```python
from build123d import *

# Parameters (mm, degrees)
CROQUIS1_W              = 400
CROQUIS1_H              = 250
SALIENTE_EXTRUIR1_DEPTH = 200
CORTAR_EXTRUIR1_DEPTH   = 115
SALIENTE_EXTRUIR2_DEPTH = 100
CHAFL_N1_SIZE           = 100
CHAFL_N1_SIZE2          = 127.994163219
CHAFL_N2_SIZE           = 127.994163219
CHAFL_N2_SIZE_2         = 100


with BuildPart() as part:
    # Croquis1 → Saliente-Extruir1 (new body)
    with BuildSketch(Plane(origin=(0, 0, 0), x_dir=(1, 0, 0), z_dir=(0, 1, 0))):
        Rectangle(CROQUIS1_W, CROQUIS1_H)
    extrude(amount=SALIENTE_EXTRUIR1_DEPTH)

    # Croquis2 → Cortar-Extruir1 (cut)
    with BuildSketch(Plane.XY.offset(125)):
        with BuildLine():
            Line((-50, 0), (50, 0))
            Line((50, 0), (50, 109.989754524))
            Line((50, 109.989754524), (49.464803301, 109.989754524))
            ThreePointArc((49.464803301, 109.989754524), (0, 159.454557825), (-49.464803301, 109.989754524))
            Line((-49.464803301, 109.989754524), (-50, 109.989754524))
            Line((-50, 109.989754524), (-50, 0))
        make_face()
    extrude(amount=-CORTAR_EXTRUIR1_DEPTH, mode=Mode.SUBTRACT)

    # Croquis4 → Saliente-Extruir2 (add)
    with BuildSketch(Plane(origin=(0, 200, 0), x_dir=(1, 0, 0), z_dir=(0, 1, 0))):
        Polygon((-200, 125), (-100, 0), (100, 0), (200, 125), align=None)
        Polygon((-100, 0), (100, 0), (200, -125), (-200, -125), align=None)
    extrude(amount=SALIENTE_EXTRUIR2_DEPTH)

    # Chaflán1
    chafl_n1_edges = [part.edges().sort_by_distance(p)[0] for p in [
        (0, 300, 125),
    ]]
    chafl_n1_side = [part.faces().sort_by_distance(p)[0] for p in [
        (0, 160.632106787, 125),
    ]]
    chamfer(chafl_n1_edges, length=CHAFL_N1_SIZE, length2=CHAFL_N1_SIZE2, reference=chafl_n1_side[0])

    # Chaflán2
    # the kernel refuses this chamfer: 127.994163219, 100 mm, written as the material it takes off along each edge
    with BuildSketch(Plane(origin=(530.165536966, 300, -125), x_dir=(0, 0.023867141339117125, 0.9997151392093142), z_dir=(-1, 0, 0))) as chafl_n2_piece_1:
        Polygon((CHAFL_N2_SIZE * 0.999715139212, -CHAFL_N2_SIZE * 0.0238671413392), (-CHAFL_N2_SIZE_2 * 0.0238671413391, -CHAFL_N2_SIZE_2 * 0.999715139209), (0, 0), align=None)
    extrude(amount=1060.331073932, mode=Mode.SUBTRACT)


solid = part.part
```
Source: CAD feature listing. Evaluate the final solid. Frame: model axes, mm. A direction names the side the tool comes from. Coordinates: 2 decimals unless noted, no trailing zeros. Write each loop counter-clockwise with the first axis right and the second up, starting at its lowest first coordinate (ties: lowest second). Pieces come first, ordered by that corner, then holes. Notation, with made-up numbers: (29, 54.5) -> (34, 54.5) arc R28 ccw to (34, 86.5) -> close; hole circle Ø7 at (25, 64.5). An arc over 180 degrees is marked (long way). Return JSON: item names as keys, results as strings. Group by question number.
1) Section query B-B, the plane z = -31. Return loops of the section in (x, y), plus the area to 3 significant figures.
2) Section query A-A, the plane x = 104.5. Return loops of the section in (y, z) (3 decimals).
3) Section query C-C, the plane x = 0. Return loops of the section in (y, z), plus the area to 3 significant figures.
4) Section query D-D, the plane z = 89. Return loops of the section in (x, y).
5) Set-up query: faces 5 (the face through (1.088, 159.443, 68.305)), 6 (the face through (160, 200, -2)), 7 (the face through (-3, 0, -2)), 8 (the face through (2.8, 238.663, 75.514)), 9 (the face through (-128.48, 226.44, -35.6)). Return all of +Z, -Z, +X, -X, +Y, -Y with unobstructed straight access to the full face (end or side cutting, diameter ignored); none if empty.
6) Mould query, pull axis Z, two halves, no side actions, for faces 1 (the face through (138.19, 237.3, 47.74)), 2 (the face through (3, 99, -125)), 3 (the face through (138.19, 237.3, -47.74)), 4 (the face through (-1, 81, 10)). Classes: +Z half, -Z half, draft (parallel to the pull), parting line (faces both ways), or undercut.
7) Ray query, line 1 along X through (y, z) = (75, 106); line 2 along Y through (x, z) = (-153.5, -34); line 3 along Z through (x, y) = (134.5, 235) (3 decimals). Return the intervals inside material, ascending.
8) Contact query for flat-ended pins moving along their axis: P1, Ø1.5, axis at y = 230.5, z = 60, coming from the -X side; P2, Ø5, axis at x = -58, z = 5, coming from the -Y side. Output: stop coordinate, or through.
From the geometry:
{
 "1": {"outline": "(-200, 0) -> (200, 0) -> (200, 200) -> (124.8, 200) -> (124.8, 273.44) -> (-124.8, 273.44) -> (-124.8, 200) -> (-200, 200) -> close", "area": "98,300 mm²"},
 "2": {"outline": "(0, -125) -> (200, -125) -> (293.266, -5.625) -> (200, -5.625) -> (200, 5.625) -> (293.266, 5.625) -> (200, 125) -> (0, 125) -> close"},
 "3": {"outline": "(0, -125) -> (200, -125) -> (297.66, 0) -> (200, 125) -> (159.45, 125) -> (159.45, 10) -> (0, 10) -> close", "area": "43,900 mm²"},
 "4": {"outline": "(-200, 0) -> (-50, 0) -> (-50, 109.99) -> (-49.46, 109.99) arc R49.46 cw to (49.46, 109.99) -> (50, 109.99) -> (50, 0) -> (200, 0) -> (200, 200) -> (171.2, 200) -> (171.2, 228.13) -> (-171.2, 228.13) -> (-171.2, 200) -> (-200, 200) -> close"},
 "5": {"face 5": "+Z, -Y", "face 6": "+X, +Y", "face 7": "+Z, -Z, +X, -X, -Y", "face 8": "+Z, +X, -X, +Y", "face 9": "-X, +Y"},
 "6": {"face 1": "undercut", "face 2": "-Z half", "face 3": "undercut", "face 4": "+Z half"},
 "7": {"line 1": "-200 to -50, 50 to 200", "line 2": "0 to 200", "line 3": "-80.202 to -43.125, 43.125 to 80.202"},
 "8": {"P1": "x = -148.6", "P2": "y = 0"}
}
